Input: part model. Units: mm. Frame: model coordinates. Face numbers are marked on the shaded views. A direction names the side the tool comes from. Coordinates: 2 decimals unless noted, no trailing zeros. Write each loop counter-clockwise with the first axis right and the second up, starting at its lowest first coordinate (ties: lowest second). Pieces come first, ordered by that corner, then holes. Notation, with made-up numbers: (9.5, 24) - (24.5, 24) arc R25 cw to (24.5, 50) - close; hole circle Ø6 at (81, 78.25). An arc over 180 degrees is marked (long way). Use a Markdown table: item, result. Add a question column.
Q1. Pin query (flat end, axial travel): P1, Ø8, axis at x = -6, y = 0.5, coming from the +Z side; P2, Ø17.5, axis at x = -1.5, z = 15, coming from the +Y side; P3, Ø8, axis at x = 2.5, y = 13.5, coming from the -Z side; P4, Ø8, axis at x = 5.5, y = 10, coming from the +Z side. Return the tip coordinate at first contact, or that it passes through.
Q2. Section query D-D (x = -6). Return the cut outline in (y, z).
Q3. Mould query, pull axis Z, two halves, no side actions, for the marked faces 1, 2, 3 and 4. Classes: released by +Z, released by -Z, zero draft, split by the parting line, or undercut.
Q4. Material intervals for probe 1 along Z at (x, y) = (-15.25, 0); probe 2 along X at (y, z) = (0, 13); probe 3 along Z at (x, y) = (-12.75, 0), sorted ascending. Write a range as from..to.
Q5. Set-up query: the marked faces 5 and 6. Return all of +Z, -Z, +X, -X, +Y, -Y with unobstructed straight access to the full face (end or side cutting, diameter ignored); none if empty.
Q6. Section query C-C (x = -15.5). Return the cut outline in (y, z).
Q7. Section query B-B (y = 23.5). Return the cut outline in (x, z), then the cut area to 3 significant figures.
Q8. Section query A-A (z = 9). Return the cut outline in (x, y).
from build123d import *

# Parameters (mm, degrees)
ESQUISSE1_W                  = 20
ESQUISSE1_H                  = 20
BOSS_EXTRU_1_DEPTH           = 24
BOSS_EXTRU_2_DEPTH           = 10
BOSS_EXTRU_2_DEPTH_BACK      = 2
ESQUISSE2_W                  = 32
ESQUISSE2_H                  = 20.000000000000448
CONG_1_R                     = 5
ENL_V_MAT_EXTRU_1_DEPTH      = 37.18550592888275
ENL_V_MAT_EXTRU_1_DEPTH_BACK = 37.18550592888275
ESQUISSE3_R                  = 7.150000000000047
CONG_4_START                 = -21
CONG_4_DEPTH                 = 31
CONG_5_R                     = 1
CONG_7_R                     = 0.25
EMPREINTE1_START             = -20
EMPREINTE1_OUTLINE_R         = 4
EMPREINTE1_DEPTH             = 8.81
ESQUISSE11_R                 = 4.150000000000001
ENL_V_MAT_EXTRU_6_DEPTH      = 8.81
CONG_20_R                    = 0.25
CONG_15_R                    = 5
ESQUISSE7_R                  = 7.4
ENL_V_MAT_EXTRU_4_DEPTH      = 37.18550609247691
BOSS_EXTRUDE1_DEPTH          = 16
CUT_EXTRUDE1_DEPTH           = 16
FILLET1_R                    = 5
FILLET2_R                    = 2
FILLET3_R                    = 1
FILLET4_R                    = 1
FILLET5_START                = 6
FILLET5_DEPTH                = 4
FILLET5_2_ANGLE              = 90
FILLET6_START                = 6
FILLET6_DEPTH                = 4
FILLET6_2_ANGLE              = 90
FILLET8_R                    = 1


with BuildPart() as part:
    # Esquisse1 → Boss.-Extru.1 (new body)
    with BuildSketch(Plane.XY):
        Rectangle(ESQUISSE1_W, ESQUISSE1_H)
    extrude(amount=BOSS_EXTRU_1_DEPTH)

    # Esquisse2 → Boss.-Extru.2 (add, two sides: drawn at the far end of the back side and taken through both)
    with BuildSketch(Plane.ZY.offset(9.999999999999998).offset(-BOSS_EXTRU_2_DEPTH_BACK)):
        with Locations((11.550204933455245, 3.980016e-11)):
            Rectangle(ESQUISSE2_W, ESQUISSE2_H)
    extrude(amount=BOSS_EXTRU_2_DEPTH + BOSS_EXTRU_2_DEPTH_BACK)

    # Congé1
    # the kernel refuses this fillet: 5 mm, written as the material it takes off along each edge
    with BuildSketch(Plane(origin=(-7.999999999999998, 22.424088128349858, -4.449795066544754), x_dir=(-1, 0, 0), z_dir=(0, -1, 0))) as cong_1_piece_1:
        with BuildLine():
            CenterArc((4.969635251323934, -5), CONG_1_R, 90, 83.68232172298448)
            Line((0, -4.449795066544754), (-0.0993927050264789, -4.438790967875649))
            ThreePointArc((-0.0993927050264789, -4.438790967875649), (-0.09999999999999964, -2.2248975332723777), (-0.09999999999999964, 0))
            Line((-0.09999999999999964, 0), (0, 0.09999999999999964))
            Line((0, 0.09999999999999964), (4.969635251323934, 0.09999999999999964))
            Line((4.969635251323934, 0.09999999999999964), (4.969635251323934, 0))
        make_face()
    extrude(amount=44.848176256620114, mode=Mode.SUBTRACT)
    with BuildSketch(Plane(origin=(-7.999999999999998, -21.962988303740985, 27.550204933455245), x_dir=(2.5e-16, 0, -1), z_dir=(0, 1, 0))) as cong_1_piece_2:
        with BuildLine():
            CenterArc((4.999999999999999, 4.785195321512226), CONG_1_R, 180, 73.1444977745706)
            Line((-1.2e-15, 4.785195321512225), (-0.10000000000000261, 4.785195321512225))
            Line((-0.10000000000000261, 4.785195321512225), (-0.10000000000000142, -3e-17))
            Line((-0.10000000000000142, -3e-17), (3e-17, -0.09999999999999964))
            ThreePointArc((3e-17, -0.09999999999999964), (1.7751024667276205, -0.0999999999999992), (3.52120903212435, -0.09570390643024408))
            Line((3.52120903212435, -0.09570390643024408), (3.5502049334552446, 0))
        make_face()
    extrude(amount=43.92597660756157, mode=Mode.SUBTRACT)

    # Esquisse3 → Enlèv. mat.-Extru.1 (cut, two sides: drawn at the far end of the back side and taken through both)
    with BuildSketch(Plane.XY.offset(24).offset(-ENL_V_MAT_EXTRU_1_DEPTH_BACK)):
        with Locations(Location((0, 0, 0), (0, 0, 180))):
            Circle(ESQUISSE3_R)
    extrude(amount=ENL_V_MAT_EXTRU_1_DEPTH + ENL_V_MAT_EXTRU_1_DEPTH_BACK, mode=Mode.SUBTRACT)

    # Congé4: read off the stored shape, not the designer's step
    # Congé4 outline → Congé4 (cut)
    with BuildSketch(Plane.YZ.offset(CONG_4_START)):
        with BuildLine():
            ThreePointArc((-5, -4.449795067), (-8.535533905, -2.985328972), (-10, 0.550204933))
            Line((-10, 0.550204933), (-10, -4.449795067))
            Line((-10, -4.449795067), (-5, -4.449795067))
        make_face()
        with BuildLine():
            Line((-10, 27.550204933), (-10, 22.550204933))
            ThreePointArc((-10, 22.550204933), (-8.535533906, 26.085738839), (-5, 27.550204933))
            Line((-5, 27.550204933), (-10, 27.550204933))
        make_face()
        with BuildLine():
            ThreePointArc((10, 0.550204933), (8.535533905, -2.985328972), (5, -4.449795067))
            Line((5, -4.449795067), (10, -4.449795067))
            Line((10, -4.449795067), (10, 0.550204933))
        make_face()
        with BuildLine():
            Line((10, 27.550204933), (5, 27.550204933))
            ThreePointArc((5, 27.550204933), (8.535533906, 26.085738839), (10, 22.550204933))
            Line((10, 22.550204933), (10, 27.550204933))
        make_face()
    extrude(amount=CONG_4_DEPTH, mode=Mode.SUBTRACT)

    # Congé5
    cong_5_edges = [part.edges().sort_by_distance(p)[0] for p in [
        (-20, 0, -4.449795066544754),
        (-20, 0, 27.550204933455245),
        (-20, 10.000000000040023, 11.550204933),
        (-20, -9.999999999960423, 11.550204933),
        (-20, 8.535533906, 26.085738839),
        (-20, -8.535533906000001, 26.085738839),
        (-20, 8.535533905, -2.985328971999999),
        (-20, -8.535533905, -2.985328972),
    ]]
    fillet(cong_5_edges, radius=CONG_5_R)

    # Congé7
    cong_7_edges = [part.edges().sort_by_distance(p)[0] for p in [
        (7.150000000000047, -1.75e-15, 24),
        (7.150000000000047, -1.75e-15, 0),
    ]]
    fillet(cong_7_edges, radius=CONG_7_R)

    # Empreinte1: read off the stored shape, not the designer's step
    # Empreinte1 outline → Empreinte1 (cut)
    with BuildSketch(Plane.YZ.offset(EMPREINTE1_START)):
        with Locations((0, 2.285680752)):
            Circle(EMPREINTE1_OUTLINE_R)
        with Locations((0, 21.714319248)):
            Circle(EMPREINTE1_OUTLINE_R)
    extrude(amount=EMPREINTE1_DEPTH, mode=Mode.SUBTRACT)

    # Esquisse11 → Enlèv. mat.-Extru.6 (cut)
    with BuildSketch(Plane.ZY.offset(19.999999999999996)):
        with Locations((2.285680751772461, -6.103752e-11)):
            Circle(ESQUISSE11_R)
        with Locations((21.714319248000876, -5.865054e-11)):
            Circle(ESQUISSE11_R)
    extrude(amount=-ENL_V_MAT_EXTRU_6_DEPTH, mode=Mode.SUBTRACT)

    # Congé20
    cong_20_edges = [part.edges().sort_by_distance(p)[0] for p in [
        (-19.999999999999996, -6.103701e-11, -1.8643192482275404),
        (-19.999999999999996, -5.865003e-11, 17.564319248000874),
    ]]
    fillet(cong_20_edges, radius=CONG_20_R)

    # Congé15
    # the kernel refuses this fillet: 5 mm, written as the material it takes off along each edge
    with BuildSketch(Plane(origin=(10.000000000000002, -9.999999999999998, -11.949795067), x_dir=(-1, 0, 0), z_dir=(0, 0, 1))) as cong_15_piece_1:
        with BuildLine():
            CenterArc((CONG_15_R, -CONG_15_R), CONG_15_R, 90, 90)
            Line((0, -CONG_15_R), (0, 0))
            Line((0, 0), (CONG_15_R, 0))
        make_face()
    extrude(amount=47.00000000000001, mode=Mode.SUBTRACT)

    # Esquisse7 → Enlèv. mat.-Extru.4 (cut, through all)
    with BuildSketch(Plane.XY.offset(24)):
        Circle(ESQUISSE7_R)
    extrude(amount=-ENL_V_MAT_EXTRU_4_DEPTH, mode=Mode.SUBTRACT)

    # Sketch1 → Boss-Extrude1 (add)
    with BuildSketch(Plane(origin=(0, 10.000000000000002, 0), x_dir=(1, 0, 0), z_dir=(0, 1, 0))):
        Polygon((10.000000000000002, -6.5), (5.000000000000002, -6.5), (4.999999999999997, -16.5), (10.000000000000005, -16.5), align=None)
    extrude(amount=BOSS_EXTRUDE1_DEPTH)

    # Sketch2 → Cut-Extrude1 (cut)
    with BuildSketch(Plane.ZY.offset(-5.000000000000004)):
        Polygon((7.7499999999999964, 24.34), (10.249999999999995, 24.34), (10.249999999999995, 16.660000000000007), (7.749999999999998, 16.66), align=None)
        Polygon((12.749999999999998, 24.340000000000003), (15.249999999999998, 24.34), (15.25, 16.660000000000014), (12.749999999999998, 16.660000000000014), align=None)
    extrude(amount=-CUT_EXTRUDE1_DEPTH, mode=Mode.SUBTRACT)

    # Fillet1
    fillet1_edges = [part.edges().sort_by_distance(p)[0] for p in [
        (5, 10.000000000000002, 11.5),
    ]]
    fillet(fillet1_edges, radius=FILLET1_R)

    # Fillet2
    # the kernel refuses this fillet: 2 mm, written as the material it takes off along each edge
    with BuildSketch(Plane(origin=(5.0000000000000036, 26, 1.5), x_dir=(-4.4e-16, -1, 0), z_dir=(-4.4e-16, 0, 1))) as fillet2_piece_1:
        with BuildLine():
            CenterArc((FILLET2_R, FILLET2_R), FILLET2_R, 180, 90)
            Line((-8.9e-16, FILLET2_R), (0, 0))
            Line((0, 0), (FILLET2_R, 0))
        make_face()
    extrude(amount=20, mode=Mode.SUBTRACT)

    # Fillet3
    fillet3_edges = [part.edges().sort_by_distance(p)[0] for p in [
        (8.5, 26, 6.5),
        (3.535533905932739, 11.464466094107284, 6.500000000000002),
        (5.000000000000002, 19.50000000002001, 6.5),
        (5.585786437626905, 25.414213562373096, 6.5),
    ]]
    fillet(fillet3_edges, radius=FILLET3_R)

    # Fillet4
    fillet4_edges = [part.edges().sort_by_distance(p)[0] for p in [
        (3.5355339059327346, 11.464466094107284, 16.5),
        (8.500000000000004, 26, 16.5),
        (4.999999999999997, 19.50000000002001, 16.5),
        (5.585786437626905, 25.414213562373096, 16.5),
    ]]
    fillet(fillet4_edges, radius=FILLET4_R)

    # Fillet5: read off the stored shape, not the designer's step
    # Fillet5 outline → Fillet5 (add)
    with BuildSketch(Plane.YZ.offset(FILLET5_START)):
        with BuildLine():
            ThreePointArc((10, 1.5), (11.464466094, 5.035533906), (15, 6.5))
            Line((15, 6.5), (10, 6.5))
            Line((10, 6.5), (10, 1.5))
        make_face()
    extrude(amount=FILLET5_DEPTH)

    # Fillet5 2 outline → Fillet5 2 (revolve)
    with BuildSketch(Plane(origin=(6, 0, 7.5), x_dir=(-3.8e-16, 0, -1), z_dir=(1, 0, -3.8e-16))):
        with BuildLine():
            Line((1, 10), (6, 10))
            ThreePointArc((6, 10), (2.464466094, 11.464466094), (1, 15))
            Line((1, 15), (1, 10))
        make_face()
    revolve(axis=Axis((6, 0, 7.5), (0, 1, 0)), revolution_arc=FILLET5_2_ANGLE)

    # Fillet6: read off the stored shape, not the designer's step
    # Fillet6 outline → Fillet6 (add)
    with BuildSketch(Plane.YZ.offset(FILLET6_START)):
        with BuildLine():
            Line((10, 16.5), (15, 16.5))
            ThreePointArc((15, 16.5), (11.464466094, 17.964466094), (10, 21.5))
            Line((10, 21.5), (10, 16.5))
        make_face()
    extrude(amount=FILLET6_DEPTH)

    # Fillet6 2 outline → Fillet6 2 (revolve)
    with BuildSketch(Plane(origin=(6, 0, 15.5), x_dir=(-1, 0, -3.2e-16), z_dir=(3.2e-16, 0, -1))):
        with BuildLine():
            Line((1, 10), (6, 10))
            ThreePointArc((6, 10), (2.464466094, 11.464466094), (1, 15))
            Line((1, 15), (1, 10))
        make_face()
    revolve(axis=Axis((6, 0, 15.5), (0, 1, 0)), revolution_arc=FILLET6_2_ANGLE)

    # Fillet8
    fillet8_edges = [part.edges().sort_by_distance(p)[0] for p in [
        (10.000000000000002, 20, 6.5),
        (10.000000000000002, 25.707106781186546, 6.792893218813452),
        (10.000000000000004, 26, 11.5),
        (10.000000000000005, 20, 16.5),
        (10.000000000000002, 25.707106781186546, 16.207106781186546),
        (10.000000000000002, 10.000000000000002, 1.0251024665),
        (10, 11.464466094, 5.0355339059999995),
        (10, 11.464466094, 17.964466094),
        (10.000000000000002, 10.000000000000002, 22.0251024665),
        (10, 9.946007309310238, 23.28301575208052),
        (10, 9.99240304129454, 0.2746838420349517),
    ]]
    fillet(fillet8_edges, radius=FILLET8_R)


solid = part.part
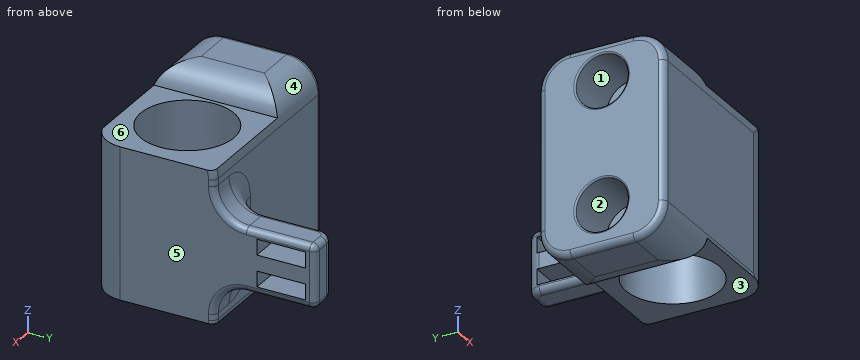
Values follow:
| question | item | result |
|---|---|---|
| 1 | P1 | z = 26.7 |
| 1 | P2 | y = 26 |
| 1 | P3 | z = 0 |
| 1 | P4 | z = 24 |
| 2 | outline | (-10, 0.55) arc R5 ccw to (-9.97, 0) - (-4.33, 0) - (-4.33, 24) - (-9.79, 24) arc R5 ccw to (-10, 22.55) - close; (4.33, 0) - (9.97, 0) arc R5 ccw to (10, 0.55) - (10, 22.55) arc R5 ccw to (9.79, 24) - (4.33, 24) - close |
| 3 | face 1 | undercut |
| 3 | face 2 | undercut |
| 3 | face 3 | released by -Z |
| 3 | face 4 | released by +Z |
| 4 | probe 1 | -4.45..-1.86, 6.44..17.56, 25.86..27.55 |
| 4 | probe 2 | -20..-7.4, 7.4..10 |
| 4 | probe 3 | -4.44..-1.86, 6.44..17.56, 25.86..27.55 |
| 5 | face 5 | +Z, -Z, +X, +Y, -Y |
| 5 | face 6 | +Z, +X, +Y, -Y |
| 6 | outline | (-10, 0.55) arc R5 ccw to (-5, -4.45) - (5, -4.45) arc R5 ccw to (10, 0.55) - (10, 22.55) arc R5 ccw to (5, 27.55) - (-5, 27.55) arc R5 ccw to (-10, 22.55) - close; hole circle Ø8.3 at (0, 2.29); hole circle Ø8.3 at (0, 21.71) |
| 7 | outline | (5, 7.5) arc R1 ccw to (6, 6.5) - (9, 6.5) arc R1 ccw to (10, 7.5) - (10, 7.75) - (5, 7.75) - close; (5, 10.25) - (10, 10.25) - (10, 12.75) - (5, 12.75) - close; (5, 15.25) - (10, 15.25) - (10, 15.5) arc R1 ccw to (9, 16.5) - (6, 16.5) arc R1 ccw to (5, 15.5) - close |
| 7 | area | 24.1 mm2 |
| 8 | outline | (-20, -9) arc R1 ccw to (-19, -10) - (5, -10) arc R5 ccw to (10, -5) - (10, 16.66) - (5, 16.66) - (5, 15) arc R5 cw to (0, 10) - (-19, 10) arc R1 ccw to (-20, 9) - close; (5.03, 24.34) - (10, 24.34) - (10, 25) arc R1 ccw to (9, 26) - (7, 26) arc R2 ccw to start; hole circle Ø14.8 at (0, 0) |
